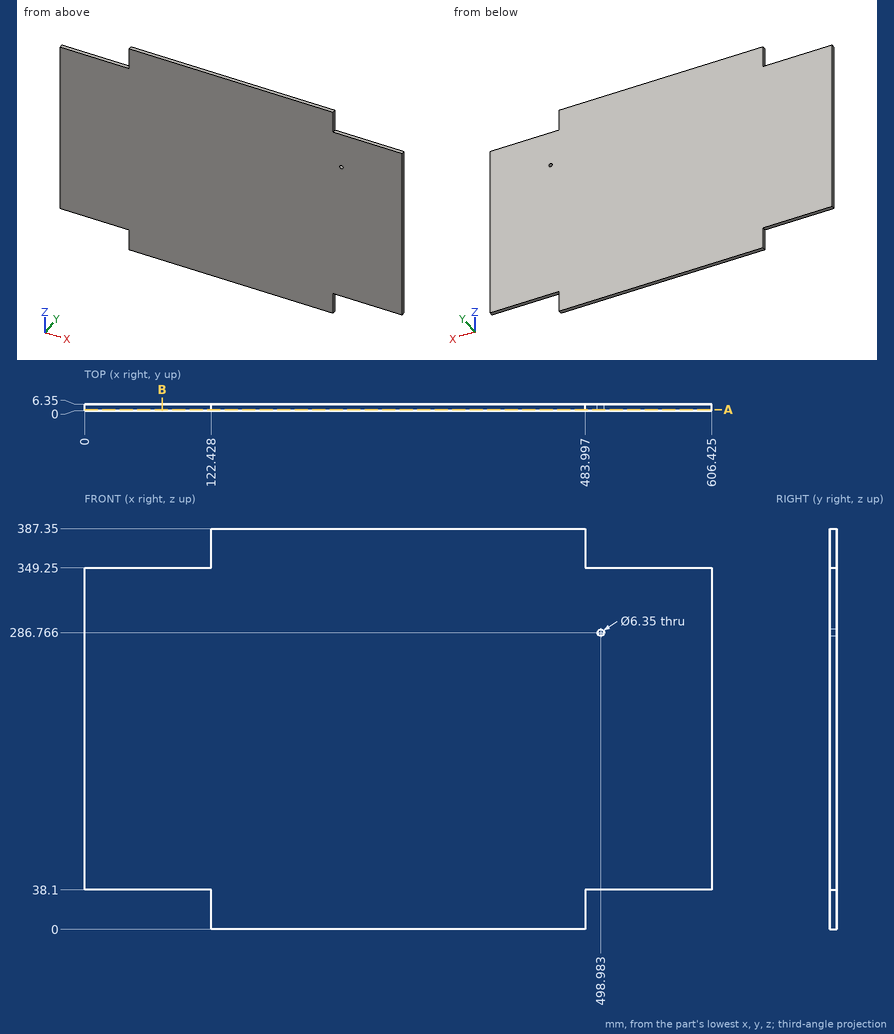
Geometry: see drawing. Coordinates: mm, zero at the bounding-box minimum. Give positions to 0.01 mm unless a question says otherwise; leave off trailing zeros. Write each loop counter-clockwise with the first axis right and the second up, starting at its lowest first coordinate (ties: lowest second). Pieces come first, ordered by that corner, then holes. Notation, with made-up numbers: M 26,-18.75 L 64,-18.75 A28 ccw 64,12.25 Z; hole C 47,86.5 d4. An arc over 180 degrees is marked long. Return JSON: item names as keys, results as strings. Group by question number.
1) Cut plane B-B, the plane x = 75. Output: boundary loops of the cut face in (y, z), then the cut area to 3 significant figures.
2) First-contact query: pin 1 Ø3 at (x, y) = (87, 4) entering from +Z; pin 2 Ø1.9 at (y, z) = (4, 13.5) entering from +X; pin 3 Ø5.5 at (x, z) = (498.983, 286.766) entering from +Y. Flat tips, straight axial feed; report the tip coordinate or a pass-through.
3) Ray query, L1, parallel to Z at x = 495.5, y = 5.75; L2, parallel to X at y = 1, z = 37. Return the intervals inside material, ascending.
4) Cut plane A-A, the plane y = 1. Output: boundary loops of the cut face in (x, z) (3 decimals).
Data:
{
 "1": {"outline": "M 0,38.1 L 6.35,38.1 L 6.35,349.25 L 0,349.25 Z", "area": "1,980 mm²"},
 "2": {"pin 1": "stops at z = 349.25", "pin 2": "stops at x = 484", "pin 3": "passes through"},
 "3": {"L1": "z = 38.1 to 349.25", "L2": "x = 122.43 to 484"},
 "4": {"outline": "M 0,38.1 L 122.428,38.1 L 122.428,0 L 483.997,0 L 483.997,38.1 L 606.425,38.1 L 606.425,349.25 L 483.997,349.25 L 483.997,387.35 L 122.428,387.35 L 122.428,349.25 L 0,349.25 Z; hole C 498.983,286.766 d6.35"}
}
